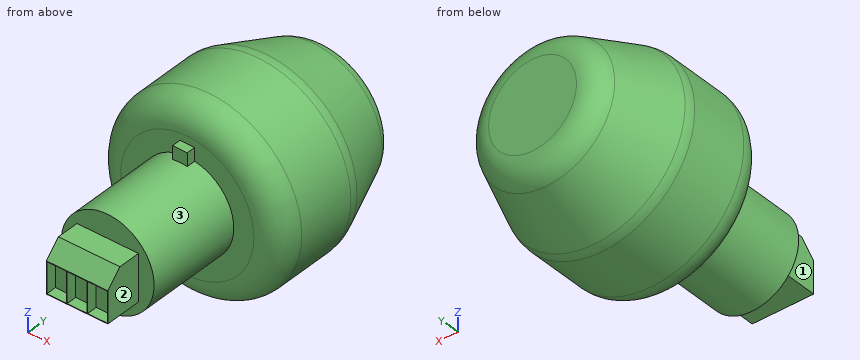
from build123d import *

# Parameters (mm, degrees)
FILLET2_R           = 6.35
BOSS_EXTRUDE1_DEPTH = 7.4549
SKETCH3_W           = 4.78028
SKETCH3_H           = 7.4422
SKETCH3_W_2         = 4.84124
CUT_EXTRUDE1_DEPTH  = 2.54
BOSS_EXTRUDE2_START = 11.097976
SKETCH4_W           = 3.556
SKETCH4_H           = 2.1844
BOSS_EXTRUDE2_DEPTH = 3.197144


with BuildPart() as part:
    # Sketch1 → Revolve1 (revolve)
    with BuildSketch(Plane.XY):
        Polygon((0, 0), (11.2395, 0), (11.2395, 23.4188), (22.473370688, 23.4188), (22.473370688, 45.4152), (14.986, 64.619312752), (0, 64.619312752), align=None)
    revolve(axis=Axis((0, 64.619312752, 0), (0, -1, 0)))

    # Fillet2
    fillet2_edges = [part.edges().sort_by_distance(p)[0] for p in [
        (-14.986, 64.619312752, 0),
        (-22.473370688, 45.4152, 0),
        (-22.473370688, 23.4188, 0),
    ]]
    fillet(fillet2_edges, radius=FILLET2_R)

    # Sketch2 → Boss-Extrude1 (add, symmetric)
    with BuildSketch(Plane(origin=(0, 0, 0), x_dir=(0, 0, -1), z_dir=(1, 0, 0))):
        Polygon((-5.626190712, 0), (5.626190712, 0), (5.626190712, -9.017181424), (-2.070009288, -9.017181424), (-5.626190712, -5.461), align=None)
    extrude(amount=BOSS_EXTRUDE1_DEPTH, both=True)

    # Sketch3 → Cut-Extrude1 (cut)
    with BuildSketch(Plane.XZ.offset(9.017181424)):
        with Locations((-4.93776, -1.778090712)):
            Rectangle(SKETCH3_W, SKETCH3_H)
        with Locations((0, -1.778090712)):
            Rectangle(SKETCH3_W_2, SKETCH3_H)
        with Locations((4.93776, -1.778090712)):
            Rectangle(SKETCH3_W, SKETCH3_H)
    extrude(amount=-CUT_EXTRUDE1_DEPTH, mode=Mode.SUBTRACT)

    # Sketch4 → Boss-Extrude2 (add)
    with BuildSketch(Plane.XY.offset(BOSS_EXTRUDE2_START)):
        with Locations((0, 22.3266)):
            Rectangle(SKETCH4_W, SKETCH4_H)
    extrude(amount=BOSS_EXTRUDE2_DEPTH)


solid = part.part
The listing builds one solid part. Answer for the finished solid, in the listing's coordinates (mm). Face numbers are marked on the shaded views. A direction names the side the tool comes from. Coordinates: 2 decimals unless noted, no trailing zeros. Loops run counter-clockwise (first coordinate to the right, second up) from the corner with the lowest first, then second, coordinate; pieces in that order, holes last. Notation, with made-up numbers: (-33.5, 3) -> (8.5, 3) arc R7 ccw to (8.5, 9) -> close; hole circle Ø7 at (-32, 83). An arc over 180 degrees is marked (long way). Write item = value, one per line. Start each with the question number.
1) A cutting plane is placed at C-C (y = -1.5). Give the vertices of the cut face in (x, z), then the cut area to 3 significant figures.
2) A cutting plane is placed at A-A (y = 39). Give the vertices of the cut face in (x, z).
3) Given pin 1 Ø1.7 at (x, y) = (-0.5, 22) entering from +Z; pin 2 Ø6 at (x, z) = (-1, -12.5) entering from -Y; pin 3 Ø2 at (y, z) = (-7.5, -0.5) entering from -X, each flat-ended and moving along its own axis, determine where each tip first touches the part or whether it passes through.
4) Straight lines are drawn through the part: line 1 (Y direction, x = -9, z = 4); line 2 (Z direction, x = 17.5, y = 44); line 3 (Z direction, x = 16.5, y = 50). For each, find the intervals that lie inside material, in ascending order. Write a range as from..to.
5) A tool of negligible diameter and unlimited length cuts with its end or side. For the marked faces 1, 2 and 3, from which of +Z, -Z, +X, -X, +Y, -Y can it reach the whole face along a straight path? Write none if from no direction.
6) A cutting plane is placed at B-B (y = 10). Give the vertices of the cut face in (x, z), then the cut area to 3 significant figures.
Responses:
q1.outline = (-7.45, -5.63) -> (7.45, -5.63) -> (7.45, 5.63) -> (-7.45, 5.63) -> close
q1.area = 168 mm²
q2.outline = circle Ø44.95 at (0, 0)
q3.pin_1 = 14.3
q3.pin_2 = 0
q3.pin_3 = -7.45
q4.line_1 = 0..64.62
q4.line_2 = -14.1..14.1
q4.line_3 = -12.48..12.48
q5.face_1 = +Z, -Z, -X, -Y
q5.face_2 = +Z, -Z, +X, -Y
q5.face_3 = -Y
q6.outline = circle Ø22.48 at (0, 0)
q6.area = 397 mm²
